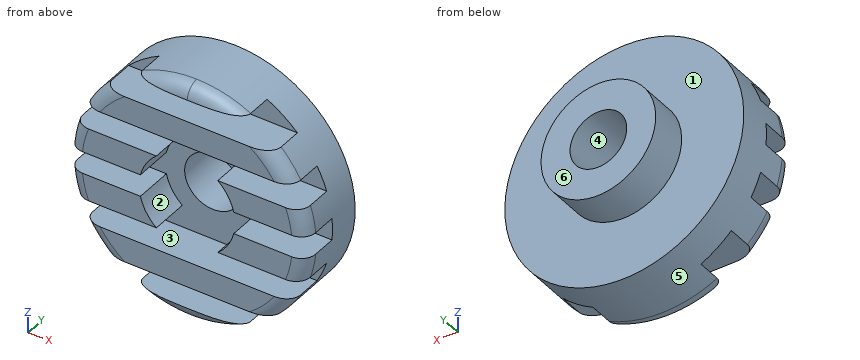
```python
from build123d import *

# Parameters (mm, degrees)
SKETCH1_R             = 25
BOSS_EXTRUDE1_DEPTH   = 15
SKETCH14_W            = 53.859934174
SKETCH14_H            = 4.599425072
CUT_EXTRUDE13_DEPTH   = 8
LPATTERN11_COUNT      = 4
LPATTERN11_PITCH      = 10
LPATTERN11_COUNT_DIR2 = 4
LPATTERN11_PITCH_DIR2 = 10
SKETCH18_R            = 10.031636401
CUT_EXTRUDE15_DEPTH   = 8
SKETCH16_R            = 12
BOSS_EXTRUDE3_DEPTH   = 8
SKETCH19_R            = 5.934931829
CUT_EXTRUDE16_DEPTH   = 26
FILLET2_R             = 3
FILLET3_R             = 3


with BuildPart() as part:
    # Sketch1 → Boss-Extrude1 (new body)
    with BuildSketch(Plane(origin=(0, 0, 0), x_dir=(1, 0, 0), z_dir=(0, 1, 0))):
        with Locations(Location((0, 0, 0), (0, 0, 270))):
            Circle(SKETCH1_R)
    extrude(amount=BOSS_EXTRUDE1_DEPTH)

    # Sketch14 → Cut-Extrude13 (cut)
    with BuildSketch(Plane(origin=(0, 0, 0), x_dir=(1, 0, 0), z_dir=(0, 1, 0))):
        Rectangle(SKETCH14_W, SKETCH14_H)
    cut_extrude13 = extrude(amount=CUT_EXTRUDE13_DEPTH, mode=Mode.SUBTRACT)

    # LPattern11: Cut-Extrude13 4 × 4
    with Locations(*[Vector(0, 0, 1) * (i * LPATTERN11_PITCH) + Vector(0, 0, -1) * (j * LPATTERN11_PITCH_DIR2) for i in range(LPATTERN11_COUNT) for j in range(LPATTERN11_COUNT_DIR2) if (i, j) != (0, 0)]):
        add(cut_extrude13, mode=Mode.SUBTRACT)

    # Sketch18 → Cut-Extrude15 (cut)
    with BuildSketch(Plane.XZ):
        Circle(SKETCH18_R)
    extrude(amount=-CUT_EXTRUDE15_DEPTH, mode=Mode.SUBTRACT)

    # Sketch16 → Boss-Extrude3 (add)
    with BuildSketch(Plane(origin=(0, 15, 0), x_dir=(1, 0, 0), z_dir=(0, 1, 0))):
        with Locations(Location((0, 0, 0), (0, 0, 270))):
            Circle(SKETCH16_R)
    extrude(amount=BOSS_EXTRUDE3_DEPTH)

    # Sketch19 → Cut-Extrude16 (cut)
    with BuildSketch(Plane(origin=(0, 23, 0), x_dir=(1, 0, 0), z_dir=(0, 1, 0))):
        with Locations(Location((0, 0, 0), (0, 0, 270))):
            Circle(SKETCH19_R)
    extrude(amount=-CUT_EXTRUDE16_DEPTH, mode=Mode.SUBTRACT)

    # Fillet2
    # the kernel refuses this fillet: 3 mm, written as the material it takes off along each edge
    with BuildSketch(Plane(origin=(0, 0, 0), x_dir=(0, 0, 1), z_dir=(-1, 0, 0))) as fillet2_piece_1_section:
        with BuildLine():
            CenterArc((25 - FILLET2_R, FILLET2_R), FILLET2_R, 270, 90)
            Line((25 - FILLET2_R, 0), (25, 0))
            Line((25, 0), (25, FILLET2_R))
        make_face()
    fillet2_piece_1 = revolve(axis=Axis((0, 0, 0), (0, 1, 0)), revolution_arc=44.06515492, mode=Mode.PRIVATE)
    fillet2_piece_1 = split(fillet2_piece_1, bisect_by=Plane(origin=(5.02070906, 0.724658167, 17.700287464), z_dir=(0, 0, 1)), keep=Keep.TOP, mode=Mode.PRIVATE)
    add(fillet2_piece_1, mode=Mode.SUBTRACT)
    with BuildSketch(Plane(origin=(0, 0, 0), x_dir=(-0.6954759312446767, 0, 0.7185493922197345), z_dir=(-0.7185493922197345, 0, -0.6954759312446767))) as fillet2_piece_2_section:
        with BuildLine():
            CenterArc((25 - FILLET2_R, FILLET2_R), FILLET2_R, 270, 90)
            Line((25 - FILLET2_R, 0), (25, 0))
            Line((25, 0), (25, FILLET2_R))
        make_face()
    fillet2_piece_2 = revolve(axis=Axis((0, 0, 0), (0, 1, 0)), revolution_arc=44.06515492, mode=Mode.PRIVATE)
    fillet2_piece_2 = split(fillet2_piece_2, bisect_by=Plane(origin=(-5.02071043, 0.724658948, 17.700287464), z_dir=(0, 0, 1)), keep=Keep.TOP, mode=Mode.PRIVATE)
    add(fillet2_piece_2, mode=Mode.SUBTRACT)

    # Fillet3
    # the kernel refuses this fillet: 3 mm, written as the material it takes off along each edge
    with BuildSketch(Plane(origin=(0, 0, 0), x_dir=(0.6954990930978064, 0, -0.7185269733977484), z_dir=(0.7185269733977484, 0, 0.6954990930978064))) as fillet3_piece_1:
        with BuildLine():
            CenterArc((25 - FILLET3_R, FILLET3_R), FILLET3_R, 270, 90)
            Line((25 - FILLET3_R, 0), (25, 0))
            Line((25, 0), (25, FILLET3_R))
        make_face()
    revolve(axis=Axis((0, 0, 0), (0, 1, 0)), revolution_arc=88.134003662, mode=Mode.SUBTRACT)
    with BuildSketch(Plane(origin=(0, 0, 0), x_dir=(0.9771108822908511, 0, -0.21273063650728477), z_dir=(0.21273063650728477, 0, 0.9771108822908511))) as fillet3_piece_2:
        with BuildLine():
            CenterArc((25 - FILLET3_R, FILLET3_R), FILLET3_R, 270, 90)
            Line((25 - FILLET3_R, 0), (25, 0))
            Line((25, 0), (25, FILLET3_R))
        make_face()
    revolve(axis=Axis((0, 0, 0), (0, 1, 0)), revolution_arc=49.979873443, mode=Mode.SUBTRACT)
    with BuildSketch(Plane(origin=(0, 0, 0), x_dir=(-0.46542458400640074, 0, -0.8850875417733937), z_dir=(0.8850875417733937, 0, -0.46542458400640074))) as fillet3_piece_3:
        with BuildLine():
            CenterArc((25 - FILLET3_R, FILLET3_R), FILLET3_R, 270, 90)
            Line((25 - FILLET3_R, 0), (25, 0))
            Line((25, 0), (25, FILLET3_R))
        make_face()
    revolve(axis=Axis((0, 0, 0), (0, 1, 0)), revolution_arc=49.979873443, mode=Mode.SUBTRACT)
    with BuildSketch(Plane(origin=(0, 0, 0), x_dir=(0.9784698974402165, 0, 0.20638958259401557), z_dir=(-0.20638958259401557, 0, 0.9784698974402165))) as fillet3_piece_4:
        with BuildLine():
            CenterArc((25 - FILLET3_R, FILLET3_R), FILLET3_R, 270, 90)
            Line((25 - FILLET3_R, 0), (25, 0))
            Line((25, 0), (25, FILLET3_R))
        make_face()
    revolve(axis=Axis((0, 0, 0), (0, 1, 0)), revolution_arc=47.03916142, mode=Mode.SUBTRACT)
    with BuildSketch(Plane(origin=(0, 0, 0), x_dir=(-0.8178655518658356, 0, -0.5754093665132607), z_dir=(0.5754093665132607, 0, -0.8178655518658356))) as fillet3_piece_5:
        with BuildLine():
            CenterArc((25 - FILLET3_R, FILLET3_R), FILLET3_R, 270, 90)
            Line((25 - FILLET3_R, 0), (25, 0))
            Line((25, 0), (25, FILLET3_R))
        make_face()
    revolve(axis=Axis((0, 0, 0), (0, 1, 0)), revolution_arc=47.03916142, mode=Mode.SUBTRACT)
    with BuildSketch(Plane(origin=(0, 0, 0), x_dir=(0.8178655518658215, 0, 0.5754093665132807), z_dir=(-0.5754093665132807, 0, 0.8178655518658215))) as fillet3_piece_6:
        with BuildLine():
            CenterArc((25 - FILLET3_R, FILLET3_R), FILLET3_R, 270, 90)
            Line((25 - FILLET3_R, 0), (25, 0))
            Line((25, 0), (25, FILLET3_R))
        make_face()
    revolve(axis=Axis((0, 0, 0), (0, 1, 0)), revolution_arc=47.03916142, mode=Mode.SUBTRACT)
    with BuildSketch(Plane(origin=(0, 0, 0), x_dir=(-0.9784698974402178, 0, -0.20638958259400958), z_dir=(0.20638958259400958, 0, -0.9784698974402178))) as fillet3_piece_7:
        with BuildLine():
            CenterArc((25 - FILLET3_R, FILLET3_R), FILLET3_R, 270, 90)
            Line((25 - FILLET3_R, 0), (25, 0))
            Line((25, 0), (25, FILLET3_R))
        make_face()
    revolve(axis=Axis((0, 0, 0), (0, 1, 0)), revolution_arc=47.03916142, mode=Mode.SUBTRACT)
    with BuildSketch(Plane(origin=(0, 0, 0), x_dir=(0.4654245840063838, 0, 0.8850875417734027), z_dir=(-0.8850875417734027, 0, 0.4654245840063838))) as fillet3_piece_8:
        with BuildLine():
            CenterArc((25 - FILLET3_R, FILLET3_R), FILLET3_R, 270, 90)
            Line((25 - FILLET3_R, 0), (25, 0))
            Line((25, 0), (25, FILLET3_R))
        make_face()
    revolve(axis=Axis((0, 0, 0), (0, 1, 0)), revolution_arc=49.979873443, mode=Mode.SUBTRACT)
    with BuildSketch(Plane(origin=(0, 0, 0), x_dir=(-0.9771108822908537, 0, 0.2127306365072725), z_dir=(-0.2127306365072725, 0, -0.9771108822908537))) as fillet3_piece_9:
        with BuildLine():
            CenterArc((25 - FILLET3_R, FILLET3_R), FILLET3_R, 270, 90)
            Line((25 - FILLET3_R, 0), (25, 0))
            Line((25, 0), (25, FILLET3_R))
        make_face()
    revolve(axis=Axis((0, 0, 0), (0, 1, 0)), revolution_arc=49.979873443, mode=Mode.SUBTRACT)


solid = part.part
```
Can you work these out from the model? Positions are in its coordinate system, mm. Face numbers are marked on the shaded views. A direction names the side the tool comes from. Coordinates: 2 decimals unless noted, no trailing zeros. Loops run counter-clockwise (first coordinate to the right, second up) from the corner with the lowest first, then second, coordinate; pieces in that order, holes last.
Item 1: Suppose I cut it at A-A (z = 0). Please give me the cut outline in (x, y), then the cut area to 3 significant figures.
Answers below:
outline: (-25, 8) - (-5.93, 8) - (-5.93, 23) - (-12, 23) - (-12, 15) - (-25, 15) - close; (5.93, 8) - (25, 8) - (25, 15) - (12, 15) - (12, 23) - (5.93, 23) - close
area: 364 mm2
Item 2: Which directions (+Z, -Z, +X, -X, +Y, -Y) give clear straight access to the entire face, cutting with the end or side of a thin tool? Please do the marked faces 1, 2 and 3.
Answers below:
face 1: +Y
face 2: -Y
face 3: +X, -X, -Y
Item 3: Please list where these lines run through material, in increasing order: L1, parallel to Z at x = 7, y = 5; L2, parallel to Z at x = 19.5, y = 6.5; L3, parallel to Y at x = 21.5, z = -8.
Answers below:
L1: z = -24 to -22.3, -17.7 to -12.3, -7.7 to -7.19, 7.19 to 7.7, 12.3 to 17.7, 22.3 to 24
L2: z = -15.64 to -12.3, -7.7 to -2.3, 2.3 to 7.7, 12.3 to 15.64
L3: y = 8 to 15
Item 4: If we mould it in two halves opening along X, with no side actions, what happens to the marked faces 4, 5 and 6? For each: released by +X, released by -X, zero draft, split by the parting line, or undercut.
Answers below:
face 4: undercut
face 5: split by the parting line
face 6: zero draft
Item 5: Suppose I cut it at B-B (y = 17.5). Please give me the cut outline in (x, z).
Answers below:
outline: circle Ø24 at (0, 0); hole circle Ø11.87 at (0, 0)
Item 6: I'm going to push flat-ended pins straight in: pin 1 (9 mm diameter, centred on x = 19, y = 2, fed in from +Z); pin 2 (6.5 mm diameter, centred on x = 3.5, y = 5, fed in from -Z); pin 3 (10 mm diameter, centred on y = 12.5, z = -12, fed in from +X). Where does each tip first touch, or does it pass through?
Answers below:
pin 1: stops at z = 17.7
pin 2: stops at z = -25
pin 3: stops at x = 24
